The model under review builds one solid part; all positions refer to its coordinate system, in mm. Face numbers are marked on the shaded views. A direction names the side the tool comes from. Round coordinates to 2 decimals unless told otherwise and drop trailing zeros. Loops run counter-clockwise (first coordinate to the right, second up) from the corner with the lowest first, then second, coordinate; pieces in that order, holes last. Notation, with made-up numbers: (-2.5, 25.5) -> (44.5, 25.5) arc R19 cw to (44.5, 37.5) -> close; hole circle Ø11 at (8, -27). An arc over 180 degrees is marked (long way). Write each question's results on one line, items separated by ' | '. Start each with the question number.
Item 1: Tool access review of the marked faces 4 and 5: name each direction out of +Z, -Z, +X, -X, +Y, -Y from which nothing blocks a thin tool from reaching the whole face with its end or side.
Item 2: We need section C-C (x = 0). Give the boundary of the cut face in (y, z), and give its area (3 significant figures).
Item 3: We need section A-A (z = 25). Give the boundary of the cut face in (x, y).
Item 4: For L1, parallel to Y at x = -9, z = -29; L2, parallel to X at y = -16.5, z = 28; L3, parallel to Y at x = -39, z = -30, list the stretches that pass through material, from the lowest coordinate up. Write a range as from..to.
Item 5: Mouldability with a two-part tool opening along X and no side actions: class the marked faces 1, 2 and 3 as pulls with the +X half, pulls with the -X half, needs draft (parallel to the pull), parting line crosses it, or undercut.
Item 6: We need section D-D (z = -11.5). Give the boundary of the cut face in (x, y).
Item 7: We need section B-B (y = 0). Give the boundary of the cut face in (x, z), and give its area (3 significant figures).
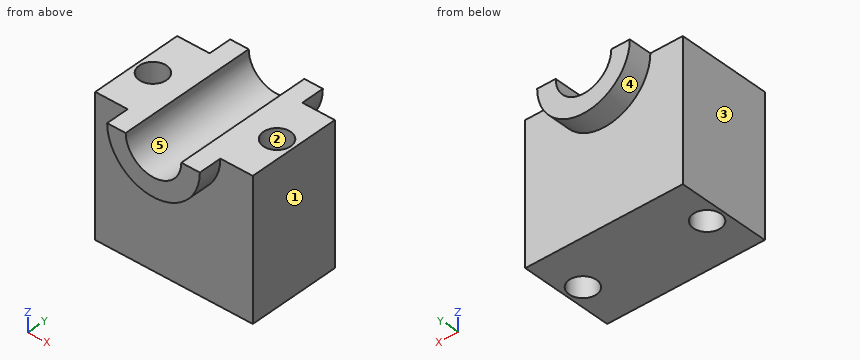
from build123d import *

# Parameters (mm, degrees)
F1_DEPTH = 38.1
F2_R     = 25.4
F2_R_2   = 15.24
F3_DEPTH = 38.1
F4_R     = 15.24
F5_DEPTH = 127
F7_DEPTH = 63.5
F8_R     = 7.4934659192
F9_DEPTH = 76.201


with BuildPart() as f1:
    # F0 (on Top) → F1 (new body, symmetric)
    with BuildSketch(Plane.XY):
        Polygon((-43.18, 0), (-43.18, -25.4), (-20.32, -25.4), (20.32, -25.4), (43.18, -25.4), (43.18, 0), (43.18, 25.4), (20.32, 25.4), (-20.32, 25.4), (-43.18, 25.4), align=None)
    extrude(amount=F1_DEPTH, both=True)

    # F2 (on Front) → F3 (join, symmetric)
    with BuildSketch(Plane.XZ):
        with Locations((0, 38.1)):
            Circle(F2_R)
        with Locations((0, 38.1)):
            Circle(F2_R_2, mode=Mode.SUBTRACT)
    extrude(amount=F3_DEPTH, both=True)

    # F4 (on face) → F5 (cut)
    with BuildSketch(Plane.XZ.offset(38.1)):
        with Locations((0, 38.1)):
            Circle(F4_R)
    extrude(amount=-F5_DEPTH, mode=Mode.SUBTRACT)

    # F6 (on Front) → F7 (cut, symmetric)
    with BuildSketch(Plane.XZ):
        Polygon((-46.0331514478, 71.8028391659), (-43.5670912266, 38.1), (43.5670949519, 38.1), (43.5670949519, 71.8028391659), align=None)
    extrude(amount=F7_DEPTH, both=True, mode=Mode.SUBTRACT)

    # F8 (on face) → F9 (cut, through all)
    with BuildSketch(Plane.XY.offset(38.1)):
        with Locations((-34.0202599764, 0)):
            Circle(F8_R)
        with Locations((34.0202599764, 0)):
            Circle(F8_R)
    extrude(amount=-F9_DEPTH, mode=Mode.SUBTRACT)


solid = f1.part
Here are the results:
1) face 4: -Z, +Y | face 5: +Z, +Y, -Y
2) outline: (-38.1, 12.7) -> (-25.4, 12.7) -> (-25.4, -38.1) -> (25.4, -38.1) -> (25.4, 12.7) -> (38.1, 12.7) -> (38.1, 22.86) -> (-38.1, 22.86) -> close | area: 3,350 mm2
3) outline: (-43.18, -25.4) -> (-21.76, -25.4) -> (-21.76, -38.1) -> (-7.79, -38.1) -> (-7.79, 38.1) -> (-21.76, 38.1) -> (-21.76, 25.4) -> (-43.18, 25.4) -> close; (7.79, -38.1) -> (21.76, -38.1) -> (21.76, -25.4) -> (43.18, -25.4) -> (43.18, 25.4) -> (21.76, 25.4) -> (21.76, 38.1) -> (7.79, 38.1) -> close; hole circle Ø14.99 at (-34.02, 0); hole circle Ø14.99 at (34.02, 0)
4) L1: y = -25.4..25.4 | L2: x = -43.18..-11.41, 11.41..43.18 | L3: y = -25.4..-5.6, 5.6..25.4
5) face 1: pulls with the +X half | face 2: undercut | face 3: pulls with the -X half
6) outline: (-43.18, -25.4) -> (43.18, -25.4) -> (43.18, 25.4) -> (-43.18, 25.4) -> close; hole circle Ø14.99 at (-34.02, 0); hole circle Ø14.99 at (34.02, 0)
7) outline: (-43.18, -38.1) -> (-41.51, -38.1) -> (-41.51, 38.1) -> (-43.18, 38.1) -> close; (-26.53, -38.1) -> (26.53, -38.1) -> (26.53, 38.1) -> (15.24, 38.1) arc R15.24 cw to (-15.24, 38.1) -> (-26.53, 38.1) -> close; (41.51, -38.1) -> (43.18, -38.1) -> (43.18, 38.1) -> (41.51, 38.1) -> close | area: 3,930 mm2
